Drawing for the job (mm, zero at the part's lowest x, y, z). A direction names the side the tool comes from. Give positions to 0.01 mm unless a question says otherwise; leave off trailing zeros. Write each loop counter-clockwise with the first axis right and the second up, starting at its lowest first coordinate (ties: lowest second). Pieces come first, ordered by that corner, then holes.
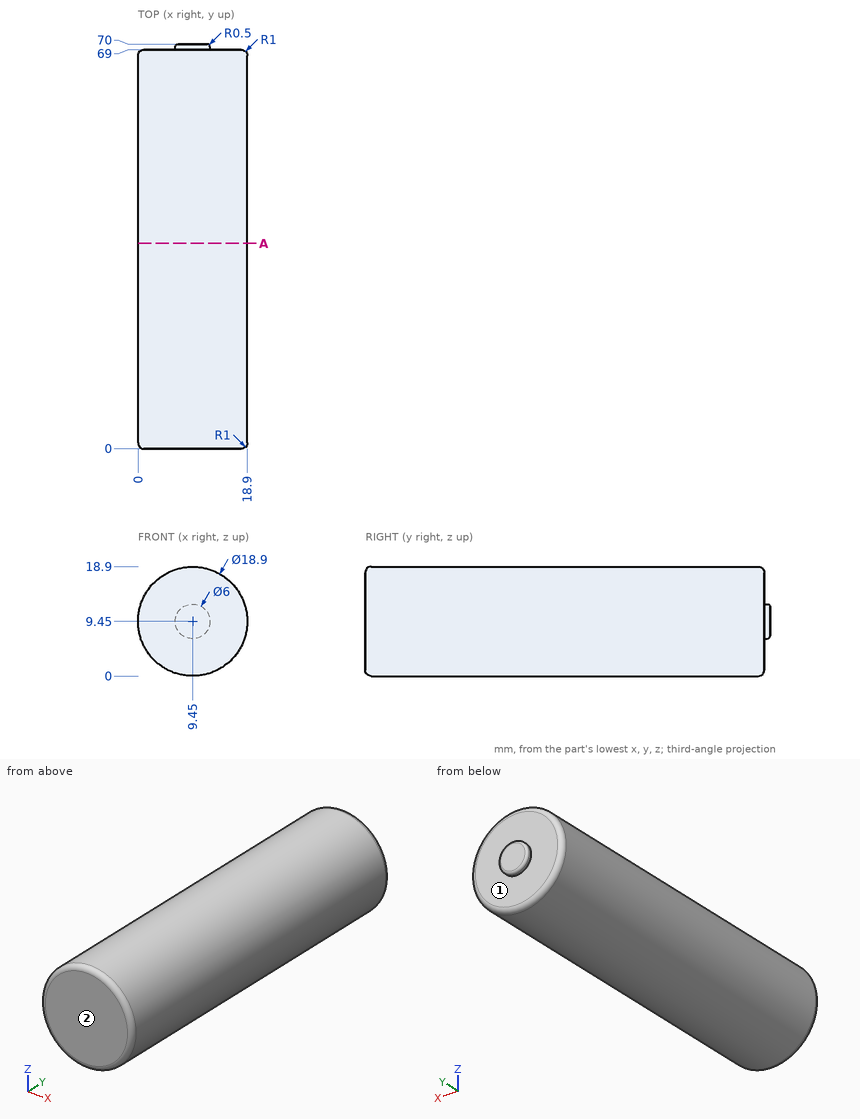
1. Slice it at A-A, the plane y = 35.5. Write the cut outline in (x, z), and give its area (3 significant figures).
Calculated:
outline: circle Ø18.9 at (9.45, 9.45)
area: 281 mm2
2. Probe probe 1 along Y at (x, z) = (1.5, 12); probe 2 along Z at (x, y) = (5.25, 7); probe 3 along X at (y, z) = (15, 11). List the from-to ranges inside material, lowest first.
Calculated:
probe 1: y = 0 to 69
probe 2: z = 0.98 to 17.92
probe 3: x = 0.13 to 18.77
3. Which spindle directions (+Z, -Z, +X, -X, +Y, -Y) get a long thin tool onto all of the face, cutting with end or side? Do the marked faces 1 and 2. Say none if no direction does.
Calculated:
face 1: +Y
face 2: +Z, -Z, +X, -X, -Y
4. Pin check, flat tips, straight feed: P1, Ø8, axis at x = 16, z = 9.5, coming from the +Y side; P2, Ø2, axis at y = 31, z = 2.5, coming from the -X side; P3, Ø4, axis at y = 28.5, z = 12.5, coming from the +X side. Stop position of each tip, or through.
Calculated:
P1: stops at y = 70
P2: stops at x = 2.11
P3: stops at x = 18.84
